Print and shaded views of the part. All mm, measured from the part's lowest x, y and z. Give positions to 0.01 mm unless a question says otherwise; leave off trailing zeros. Order: outer loops, then holes, each group sorted by start corner. A loop starts at its lowest first (then second) coordinate and runs counter-clockwise, first axis right, second up. Notation, with made-up numbers: (-4, 17) - (48, 17) arc R12 ccw to (48, 38) - close; hole circle Ø7 at (-11.5, 32.5). An arc over 180 degrees is marked (long way). Answer in a Markdown table with one row per item.
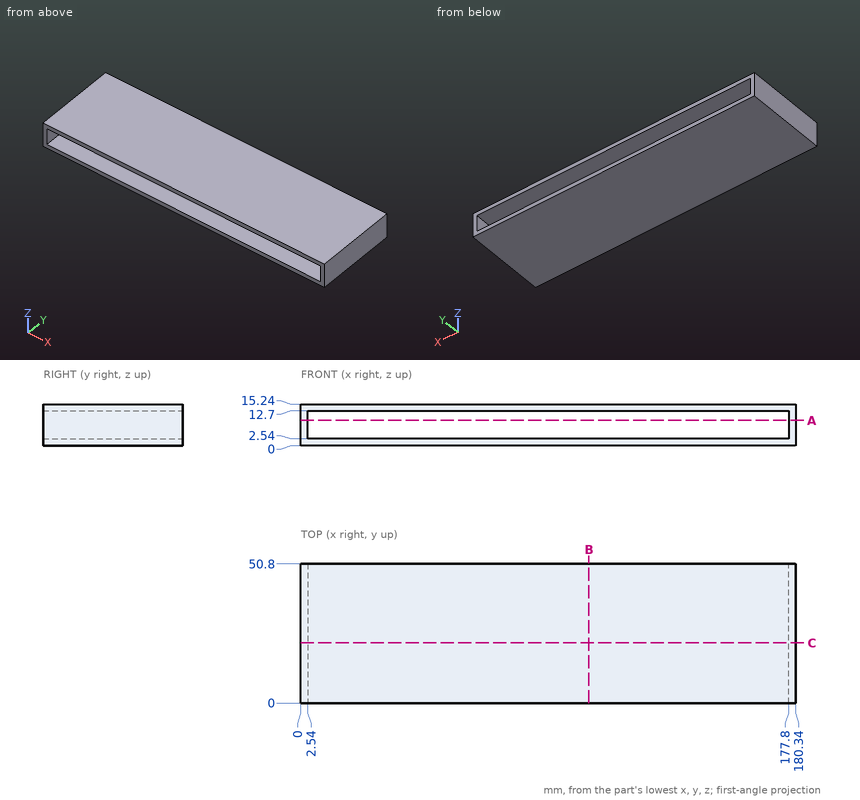
1. Cut at C-C on y = 22. Write the cut outline in (x, z), and give its area (3 significant figures).
Check result:
| item | result |
|---|---|
| outline | (0, 0) - (180.34, 0) - (180.34, 15.24) - (0, 15.24) - close; hole (2.54, 2.54) - (177.8, 2.54) - (177.8, 12.7) - (2.54, 12.7) - close |
| area | 968 mm² |
2. Cut at A-A on z = 9.25. Write the cut outline in (x, y).
Check result:
| item | result |
|---|---|
| outline | (0, 0) - (2.54, 0) - (2.54, 50.8) - (0, 50.8) - close; (177.8, 0) - (180.34, 0) - (180.34, 50.8) - (177.8, 50.8) - close |
3. Cut at B-B on x = 105. Write the cut outline in (y, z), and give its area (3 significant figures).
Check result:
| item | result |
|---|---|
| outline | (0, 0) - (50.8, 0) - (50.8, 2.54) - (0, 2.54) - close; (0, 12.7) - (50.8, 12.7) - (50.8, 15.24) - (0, 15.24) - close |
| area | 258 mm² |
4. Probe line 1 (X direction, y = 10.5, z = 8); line 2 (Z direction, x = 41, y = 45). List the from-to ranges inside material, lowest first.
Check result:
| item | result |
|---|---|
| line 1 | x = 0 to 2.54, 177.8 to 180.34 |
| line 2 | z = 0 to 2.54, 12.7 to 15.24 |
